Input: part model. Units: mm. Frame: model coordinates. A direction names the side the tool comes from. Coordinates: 2 decimals unless noted, no trailing zeros. Loops run counter-clockwise (first coordinate to the right, second up) from the corner with the lowest first, then second, coordinate; pieces in that order, holes last. Notation, with made-up numbers: M -3,33 L 54,33 A13 cw 54,57 Z; hole C -4,-13 d5. An arc over 180 degrees is marked long. Use a Markdown table: item, result. Add a question column.
1. Set-up query: faces 1 (the flat face through (-12.091, 9, -13)), 2 (the flat face through (-3.3, -15, -8)), 3 (the cylindrical face through (-9.39, 3.515, 0.271)). Return all of +Z, -Z, +X, -X, +Y, -Y with unobstructed straight access to the full face (end or side cutting, diameter ignored); none if empty.
2. Section B-B on y = 8. State how many separate pieces and enclosed holes the cut face has, then the cut area to 3 significant figures.
3. Section A-A on z = 7. Output: boundary loops of the cut face in (x, y).
4. Line query: L1, parallel to X at y = -33, z = 1.5; L2, parallel to Z at x = 4.5, y = -26.5; L3, parallel to X at y = -10.5, z = -10. Output: solid intervals per line, ascending. Write a range as [from, to].
5. Pin query (flat end, axial travel): pin 1 (12 mm diameter, centred on y = 3.5, z = 9.5, fed in from -X); pin 2 (4.5 mm diameter, centred on y = 11.5, z = 5.5, fed in from -X); pin 3 (3 mm diameter, centred on y = -50, z = 5.5, fed in from +X). Return the tip coordinate at first contact, or that it passes through.
6. Draft query along Z for faces 4 (the flat face through (-2, -3, -17.5)), 5 (the flat face through (10.909, 0, 0)), 6 (the flat face through (3.04, 7.18, 0.25)). Return one class per face: +Z half, -Z half, draft (parallel to the pull), parting line (faces both ways), or undercut.
7. Section C-C on z = -3. Output: boundary loops of the cut face in (x, y), then the cut area to 4 significant figures.
Autodesk Inventor part; units mm, degrees
ref_plane "YZ Plane" through (0, 0, 0) normal (1, 0, 0) x (0, 1, 0)
ref_plane "XZ Plane" through (0, 0, 0) normal (0, 1, 0) x (-1, 0, 0)
ref_plane "XY Plane" through (0, 0, 0) normal (0, 0, 1) x (1, 0, 0)
sketch "Sketch1" plane through (0, 0, 0) normal (0, 0, 1) x (1, 0, 0)
  line L0 (10.9091, 15) -> (-12.0909, 15)
  line L1 (-12.0909, 15) -> (-12.0909, -15)
  line L2 (-12.0909, -15) -> (10.9091, -15)
  line L3 (10.9091, -15) -> (10.9091, 15)
  line L4 (-12.0909, -15) -> (-22.6975, -4.3934)
  line L5 (-12.0909, -15) -> (2.9091, -15) construction
  line L6 (-22.6975, -4.3934) -> (-12.0909, 6.2132)
  line L7 (-12.0909, 6.2132) -> (2.0731, -7.9508) construction
  line L8 (10.9091, 15.0492) -> (-9.4479, -5.3079) construction
  line L9 (-8.4113, 37.889) -> (15.6041, 13.8735) construction
  line L10 (-5.0089, -0.8688) -> (12.6688, 16.8089)
  line L11 (12.6688, 16.8089) -> (-8.4113, 37.889)
  line L12 (-8.4113, 37.889) -> (-26.089, 20.2113)
  line L13 (-26.089, 20.2113) -> (-5.0089, -0.8688)
  point P0 (0, 0)
  point P1 (10.9091, 0)
  dimension "d0" = 30
  dimension "d1" = 23
  dimension "d2" = 15
  dimension "d3" = 135
  dimension "d4" = 15
  dimension "d5" = 25
extrude "Extrusion1" add sketch "Sketch1" along normal mid plane 35 contours L3 L2 L1 L13 L10 L0 | L10 L13 L1 L0 | L4 L6 L1
revolve "Revolution1" cut sketch "Sketch1" angle 360 about axis through (12.6688, 16.8089, 0) along (-0.7071, 0.7071, 0) contours L10 L13 L1 L0 | L0 L1 L13 L12 L11 L10
sketch "Sketch2" plane through (-12.0909, -15, 17.5) normal (0, -1, 0) x (1, 0, 0)
  circle A0 centre (12.0909, -17.5) radius 8.5
  dimension "d9" = 17
extrude "Extrusion2" add sketch "Sketch2" along normal blind 65
properties part number "Feed_pin"
Answers below:
| question | item | result |
|---|---|---|
| 1 | face 1 | +Z, -Z, -X, +Y |
| 1 | face 2 | -Y |
| 1 | face 3 | +Y |
| 2 | separate pieces | 3 |
| 2 | enclosed holes | 0 |
| 2 | area | 313 mm² |
| 3 | outline | M -22.7,-4.39 L -12.09,-15 L -4.82,-15 L -4.82,-80 L 4.82,-80 L 4.82,-15 L 10.91,-15 L 10.91,15 L 10.86,15 L -4.3,-0.16 L -12.09,7.63 L -12.09,6.21 Z |
| 4 | L1 | x = [-8.37, 8.37] |
| 4 | L2 | z = [-7.21, 7.21] |
| 4 | L3 | x = [-16.59, 10.91] |
| 5 | pin 1 | stops at x = -20.8 |
| 5 | pin 2 | stops at x = 5.11 |
| 5 | pin 3 | stops at x = 7.5 |
| 6 | face 4 | -Z half |
| 6 | face 5 | draft |
| 6 | face 6 | undercut |
| 7 | outline | M -22.7,-4.39 L -12.09,-15 L -7.95,-15 L -7.95,-80 L 7.95,-80 L 7.95,-15 L 10.91,-15 L 10.91,15 L 10.86,15 L -4.88,-0.74 L -12.09,6.47 L -12.09,6.21 Z |
| 7 | area | 1,625 mm² |
